```python
from build123d import *

# Parameters (mm, degrees)
SKETCH2_W          = 26.67
SKETCH2_H          = 26.67
SKETCH2_W_2        = 21.59
SKETCH2_H_2        = 21.59
SKETCH4_R          = 4.7625
CUT_EXTRUDE2_DEPTH = 234.463995003
SKETCH5_R          = 1.27
CUT_EXTRUDE3_DEPTH = 234.463995003


with BuildPart() as part:
    # Sweep1: sweep along a path in Sketch1
    with BuildLine(Plane.XY) as sweep1_path:
        Line((0, 0), (-171.835765676, 0))
        Line((-171.835765676, 0), (-182.88, 0))
        Line((-182.88, 0), (-190.412149697, 8.077241654))
        Line((-190.412149697, 8.077241654), (-217.525516691, 37.152768042))
    # Sketch2 → Sweep1 (sweep)
    with BuildSketch(Plane(origin=(0, 0, 0), x_dir=(0, 0, -1), z_dir=(1, 0, 0))):
        Rectangle(SKETCH2_W, SKETCH2_H)
        Rectangle(SKETCH2_W_2, SKETCH2_H_2, mode=Mode.SUBTRACT)
    sweep(path=sweep1_path.line, transition=Transition.RIGHT)

    # Sketch4 → Cut-Extrude2 (cut, through all)
    with BuildSketch(Plane.XY.offset(13.335)):
        with Locations((-33.788615372, 1.553440166)):
            Circle(SKETCH4_R)
    extrude(amount=-CUT_EXTRUDE2_DEPTH, mode=Mode.SUBTRACT)

    # Sketch5 → Cut-Extrude3 (cut, through all)
    with BuildSketch(Plane.XY.offset(13.335)):
        with Locations((-203.326149514, 23.038600359)):
            Circle(SKETCH5_R)
        with Locations((-208.411861608, 17.628386689)):
            Circle(SKETCH5_R)
    extrude(amount=-CUT_EXTRUDE3_DEPTH, mode=Mode.SUBTRACT)


solid = part.part
```
The model under review builds one solid part; all positions refer to its coordinate system, in mm. A direction names the side the tool comes from. Round coordinates to 2 decimals unless told otherwise and drop trailing zeros. Loops run counter-clockwise (first coordinate to the right, second up) from the corner with the lowest first, then second, coordinate; pieces in that order, holes last. Notation, with made-up numbers: M 33,19.5 L 71,19.5 A21 cw 71,42.5 Z; hole C -14.5,-10.75 d2. An arc over 180 degrees is marked long. Put each result on its own line as item: value.
Q1. For pin 1 (6.5 mm diameter, centred on x = -70.5, z = 1, fed in from +Y) (3 decimals); pin 2 (8 mm diameter, centred on y = 29, z = 8.5, fed in from +X); pin 3 (5 mm diameter, centred on y = -3.5, z = 8.5, fed in from -X); pin 4 (2 mm diameter, centred on x = -203.33, y = 23.04, fed in from +Z), all flat-tipped, find the tip position at first contact; note any pin that passes through.
Result set:
pin 1: stops at y = 13.335
pin 2: stops at x = -187.96
pin 3: stops at x = -200.18
pin 4: passes through
Q2. Machinability: for faces 1 (the flat face through (-90, 13.335, 0)), 2 (the flat face through (-95, -10.795, 0)), 3 (the flat face through (-114, 4, 10.795)), which of the approach directions +Z, -Z, +X, -X, +Y, -Y give a long, thin tool a straight path to every point of the face, cutting with its end or side? Answer none if there is none.
Result set:
face 1: +Z, -Z, +X, +Y
face 2: +X
face 3: none
Q3. Consider section A-A, the plane z = -7.25. Give the boundary of the cut face in (x, y) (3 decimals), then the cut area to 3 significant figures.
Result set:
outline: M -227.278,28.058 L -188.678,-13.335 L 0,-13.335 L 0,-10.795 L -187.574,-10.795 L -225.42,29.791 Z; M -209.631,44.515 L -178.186,10.795 L 0,10.795 L 0,13.335 L -177.082,13.335 L -207.773,46.247 Z
area: 1,190 mm²
Q4. Consider section C-C, the plane y = 35. Give the boundary of the cut face in (x, z) (3 decimals).
Result set:
outline: M -219.834,-13.335 L -197.285,-13.335 L -197.285,13.335 L -219.834,13.335 L -219.834,10.795 L -200.758,10.795 L -200.758,-10.795 L -219.834,-10.795 Z
Q5. Consider section B-B, the plane x = -46.5. Give the boundary of the cut face in (y, z) (3 decimals), then the cut area to 3 significant figures.
Result set:
outline: M -13.335,-13.335 L 13.335,-13.335 L 13.335,13.335 L -13.335,13.335 Z; hole M -10.795,-10.795 L 10.795,-10.795 L 10.795,10.795 L -10.795,10.795 Z
area: 245 mm²
Q6. Consider section D-D, the plane y = -6. Give the boundary of the cut face in (x, z) (3 decimals).
Result set:
outline: M -195.518,-13.335 L 0,-13.335 L 0,-10.795 L -192.045,-10.795 L -192.045,10.795 L 0,10.795 L 0,13.335 L -195.518,13.335 Z
Q7. Mouldability with a two-part tool opening along Z and no side actions: class faces 4 (the flat face through (-90, 10.795, 0)), 5 (the flat face through (-115, 3, -13.335)), 6 (the flat face through (-115, 4, 13.335)), 7 (the flat face through (-113, 5, -10.795)) as released by +Z, released by -Z, zero draft, split by the parting line, or undercut.
Result set:
face 4: undercut
face 5: released by -Z
face 6: released by +Z
face 7: undercut
Q8. To check wall thickness, follow L1, parallel to Y at x = -132, z = 10.75 (3 decimals); L2, parallel to Y at x = -169.5, z = 11 (3 decimals). State the ranges of each line that lie inside material, in increasing order.
Result set:
L1: y = -13.335 to -10.795, 10.795 to 13.335
L2: y = -13.335 to 13.335
